Autodesk Inventor part; units mm, degrees
ref_plane "YZ Plane" through (0, 0, 0) normal (1, 0, 0) x (0, 1, 0)
ref_plane "XZ Plane" through (0, 0, 0) normal (0, 1, 0) x (-1, 0, 0)
ref_plane "XY Plane" through (0, 0, 0) normal (0, 0, 1) x (1, 0, 0)
sketch "Sketch1" plane through (0, 0, 0) normal (0, 1, 0) x (-1, 0, 0)
  line L0 (0, 0) -> (33, 0)
  line L1 (33, 0) -> (33, -69)
  line L2 (33, -69) -> (0, -69)
  line L3 (2, -2) -> (31, -2)
  line L4 (31, -2) -> (31, -67)
  line L5 (31, -67) -> (2, -67)
  line L6 (2, -2) -> (0, -2)
  line L7 (2, -67) -> (0, -67)
  line L8 (0, -69) -> (0, -67)
  line L9 (0, -2) -> (0, 0)
  dimension "d0" = 2
  dimension "d1" = 2
  dimension "d3" = 2
  dimension "d4" = 33
  dimension "d5" = 69
  dimension "d7" = 0
extrude "Extrusion1" add sketch "Sketch1" along normal blind 6
sketch "Sketch2" plane through (0, 6, 0) normal (0, 1, 0) x (1, 0, 0)
  line L0 (0, 0) -> (0, 2)
  line L1 (0, 69) -> (-33, 69)
  line L2 (0, 0) -> (-33, 0)
  line L3 (-33, 0) -> (-33, 69)
  line L4 (-33, 69) -> (0, 69)
  line L5 (0, 69) -> (0, 0)
extrude "Extrusion2" add sketch "Sketch2" along normal blind 2
sketch "Sketch3" plane through (0, 8, 0) normal (0, 1, 0) x (1, 0, 0)
  circle A0 centre (-18, 15.5) radius 8
  circle A1 centre (-18, 53.5) radius 8
  line L0 (-33, 69) -> (-33, 0) construction
  line L1 (-33, 34.5) -> (0, 34.5) construction
  line L2 (0, 2) -> (0, 67) construction
  line L3 (-33, 0) -> (0, 0) construction
  dimension "d12" = 16
  dimension "d13" = 16
  dimension "d14" = 34.5
  dimension "d15" = 19
  dimension "d16" = 19
  dimension "d17" = 15
  dimension "d18" = 15
extrude "Extrusion3" cut sketch "Sketch3" against normal blind 2
sketch "Sketch4" plane through (-33, 0, -69) normal (-1, 0, 0) x (0, 0, 1)
  line L0 (67, 0) -> (2, 0)
  line L1 (27, 0) -> (42, 0)
  line L2 (42, 0) -> (42, 8)
  line L3 (42, 8) -> (27, 8)
  line L4 (27, 8) -> (27, 0)
  line L5 (0, 0) -> (0, 8)
  point P0 (69, 0)
  dimension "d21" = 15
  dimension "d22" = 27
  dimension "d23" = 8
extrude "Extrusion4" cut sketch "Sketch4" against normal blind 4
properties part number "top"
Verification items for the finished model (mm, model axes). A direction names the side the tool comes from. Coordinates: 2 decimals unless noted, no trailing zeros. Write each loop counter-clockwise with the first axis right and the second up, starting at its lowest first coordinate (ties: lowest second). Pieces come first, ordered by that corner, then holes. Notation, with made-up numbers: (-36.75, 0) - (-9.75, 0) arc R29 cw to (-9.75, 38) - close; hole circle Ø4 at (-10.5, 88.5). An arc over 180 degrees is marked (long way). Write item = value, one per line.
Q1. Cross-section at D-D (y = 7.25). Enter the section's corners in (x, z).
Answer:
outline = (-33, -69) - (0, -69) - (0, 0) - (-33, 0) - (-33, -27) - (-29, -27) - (-29, -42) - (-33, -42) - close; hole circle Ø16 at (-18, -53.5); hole circle Ø16 at (-18, -15.5)
Q2. Cross-section at C-C (x = -18). Enter the section's corners in (y, z).
Answer:
outline = (0, -69) - (8, -69) - (8, -61.5) - (6, -61.5) - (6, -67) - (0, -67) - close; (0, -2) - (6, -2) - (6, -7.5) - (8, -7.5) - (8, 0) - (0, 0) - close; (6, -45.5) - (8, -45.5) - (8, -23.5) - (6, -23.5) - close
Q3. Cross-section at A-A (y = 1.25). Enter the section's corners in (x, z).
Answer:
outline = (-33, -69) - (0, -69) - (0, -67) - (-31, -67) - (-31, -42) - (-33, -42) - close; (-33, -27) - (-31, -27) - (-31, -2) - (0, -2) - (0, 0) - (-33, 0) - close
Q4. Access from +Z, -Z, +X, -X, +Y, -Y to the whole of each face (thin tool, end or side, straight path). Record for faces 1 (the face through (-31.5, 4.9, -42)), 2 (the face through (-19.041, 7.014, -61.432)), 3 (the face through (-16, 3, -67)).
Answer:
face_1 = -X, +Y, -Y
face_2 = +Y, -Y
face_3 = +X, -Y
Q5. Cross-section at B-B (z = -15.5). Enter the section's corners in (x, y), plus the area to 3 significant figures.
Answer:
outline = (-33, 0) - (-31, 0) - (-31, 6) - (-26, 6) - (-26, 8) - (-33, 8) - close; (-10, 6) - (0, 6) - (0, 8) - (-10, 8) - close
area = 46.0 mm²
Q6. Mould release check, pull along Z, two halves, no side actions. Record for faces 4 (the face through (-24.349, 7.014, -10.632)), 5 (the face through (-24, 0, -1)), 6 (the face through (-17, 4, -69)): released by +Z, released by -Z, zero draft, split by the parting line, or undercut.
Answer:
face_4 = undercut
face_5 = zero draft
face_6 = released by -Z
Q7. Material ranges on L1, parallel to Z at x = -18, y = 7.5; L2, parallel to X at y = 7, z = -53.5; L3, parallel to Z at x = -21, y = 7.5, recorded low to high. Write a range as from..to.
Answer:
L1 = -69..-61.5, -45.5..-23.5, -7.5..0
L2 = -33..-26, -10..0
L3 = -69..-60.92, -46.08..-22.92, -8.08..0
Q8. Go/stop test with flat-tipped pins: pin 1 Ø3 at (y, z) = (3, -12.5) entering from +X; pin 2 Ø18.5 at (x, z) = (-18, -15.5) entering from -Y; pin 3 Ø1 at (y, z) = (6.5, -32.5) entering from -X. Record where each tip stops, or that it passes through.
Answer:
pin_1 = -31
pin_2 = 6
pin_3 = -29
